CAD build for the part. Positions are in the model's coordinates, mm. Give positions to 0.01 mm unless a question says otherwise; leave off trailing zeros. Order: outer loops, then holes, each group sorted by start corner. A loop starts at its lowest first (then second) coordinate and runs counter-clockwise, first axis right, second up.
Item 1: Band-saw the part on B-B on y = 0. Give the cut face in (x, z).
Item 2: Band-saw the part on A-A on x = 0. Count the separate pieces of the cut face and the enclosed holes in it, plus the area to 3 significant figures.
Item 3: Wall check: L1, parallel to Y at x = 0, z = -25.7; L2, parallel to Y at x = -1, z = -27.75; L3, parallel to Y at x = -14.5, z = -27.25. Give the ranges that are in metal, low to high.
Item 4: Flat gauge pins, fed straight in: P1, Ø3, axis at x = -28.58, y = -16.5, coming from the -Z side; P2, Ø1.5, axis at y = -28, z = -25.5, coming from the -X side; P3, Ø3.5, axis at x = 0, y = -33, coming from the -Z side; P4, Ø2, axis at x = -28.5, z = -28.5, coming from the +Y side. Where does each tip first touch, or does it go through?
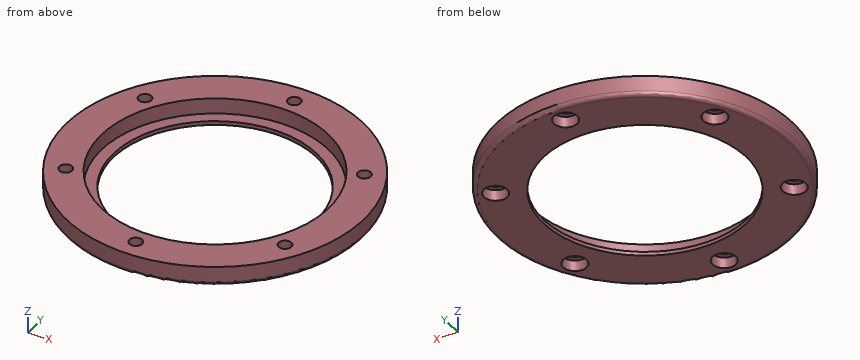
```python
from build123d import *

# Parameters (mm, degrees)
SKETCH_1_W                    = 38
SKETCH_1_H                    = 5
HOLE_WIZARD_M48_1_D           = 52
HOLE_WIZARD_M48_1_DEPTH       = 5
HOLE_WIZARD_M48_1_CBORE_D     = 58.1
HOLE_WIZARD_M48_1_CBORE_DEPTH = 4
SKETCH_16_R                   = 1.65
CUT_EXTRUDE_9_DEPTH           = 6
SKETCH_17_R                   = 3
CUT_EXTRUDE_10_DEPTH          = 2.8
FILLET_2_R                    = 1


with BuildPart() as part:
    # 草图1 → 旋转1 (revolve)
    with BuildSketch(Plane(origin=(0, 0, 0), x_dir=(1, 0, 0), z_dir=(0, 1, 0))):
        with Locations((19, 26.5)):
            Rectangle(SKETCH_1_W, SKETCH_1_H)
    revolve(axis=Axis((0, 0, -29), (0, 0, 1)))

    # M48 六角头螺栓的柱形沉头孔1
    with Locations(Plane.XY.offset(-24)):
        with Locations((0, 0)):
            CounterBoreHole(HOLE_WIZARD_M48_1_D / 2, HOLE_WIZARD_M48_1_CBORE_D / 2, HOLE_WIZARD_M48_1_CBORE_DEPTH, depth=HOLE_WIZARD_M48_1_DEPTH)

    # 草图16 → 切除-拉伸9 (cut, through all)
    with BuildSketch(Plane(origin=(0, 0, -29), x_dir=(-1, 0, 0), z_dir=(0, 0, -1))):
        with Locations((0, -33)):
            Circle(SKETCH_16_R)
        with Locations((-28.578838325, -16.5)):
            Circle(SKETCH_16_R)
        with Locations((-28.578838325, 16.5)):
            Circle(SKETCH_16_R)
        with Locations((0, 33)):
            Circle(SKETCH_16_R)
        with Locations((28.578838325, 16.5)):
            Circle(SKETCH_16_R)
        with Locations((28.578838325, -16.5)):
            Circle(SKETCH_16_R)
    extrude(amount=-CUT_EXTRUDE_9_DEPTH, mode=Mode.SUBTRACT)

    # 草图17 → 切除-拉伸10 (cut)
    with BuildSketch(Plane(origin=(0, 0, -29), x_dir=(-1, 0, 0), z_dir=(0, 0, -1))):
        with Locations((0, -33)):
            Circle(SKETCH_17_R)
        with Locations((-28.578838325, -16.5)):
            Circle(SKETCH_17_R)
        with Locations((-28.578838325, 16.5)):
            Circle(SKETCH_17_R)
        with Locations((0, 33)):
            Circle(SKETCH_17_R)
        with Locations((28.578838325, 16.5)):
            Circle(SKETCH_17_R)
        with Locations((28.578838325, -16.5)):
            Circle(SKETCH_17_R)
    extrude(amount=-CUT_EXTRUDE_10_DEPTH, mode=Mode.SUBTRACT)

    # 圆角2
    fillet_2_edges = [part.edges().sort_by_distance(p)[0] for p in [
        (-38, 0, -29),
    ]]
    fillet(fillet_2_edges, radius=FILLET_2_R)


solid = part.part
```
The answers:
1. outline: (-38, -28) arc R1 ccw to (-37, -29) - (-26, -29) - (-26, -28) - (-29.05, -28) - (-29.05, -24) - (-38, -24) - close; (26, -29) - (37, -29) arc R1 ccw to (38, -28) - (38, -24) - (29.05, -24) - (29.05, -28) - (26, -28) - close
2. separate pieces: 4
2. enclosed holes: 0
2. area: 47.1 mm2
3. L1: y = -38 to -34.65, -31.35 to -29.05, 29.05 to 31.35, 34.65 to 38
3. L2: y = -37.99 to -35.83, -30.17 to -29.03, 29.03 to 30.17, 35.83 to 37.99
3. L3: y = -35.12 to -25.17, 25.17 to 35.12
4. P1: passes through
4. P2: stops at x = -26.48
4. P3: stops at z = -26.2
4. P4: stops at y = 26.15
